Read the model definition and answer for the solid it produces. Units are mm, in the model's axes. Give positions to 0.01 mm unless a question says otherwise; leave off trailing zeros. Write each loop counter-clockwise with the first axis right and the second up, starting at its lowest first coordinate (ties: lowest second). Pieces come first, ordered by that corner, then holes.
```python
from build123d import *

# Parameters (mm, degrees)
SKETCH1_W           = 25.4
SKETCH1_H           = 25.4
SKETCH1_W_2         = 20.32
SKETCH1_H_2         = 20.32
BOSS_EXTRUDE2_DEPTH = 368.3
CUT_EXTRUDE1_DEPTH  = 370.393205135
SKETCH3_R           = 3.175
CUT_EXTRUDE2_DEPTH  = 370.393205135


with BuildPart() as part:
    # Sketch1 → Boss-Extrude2 (new body)
    with BuildSketch(Plane.XY):
        Rectangle(SKETCH1_W, SKETCH1_H)
        Rectangle(SKETCH1_W_2, SKETCH1_H_2, mode=Mode.SUBTRACT)
    extrude(amount=BOSS_EXTRUDE2_DEPTH)

    # Sketch2 → Cut-Extrude1 (cut, through all)
    with BuildSketch(Plane(origin=(0, 12.7, 0), x_dir=(1, 0, 0), z_dir=(0, 1, 0))):
        Polygon((-12.7, -368.3), (12.7, -353.635303163), (12.7, -368.3), align=None)
        Polygon((12.7, 0), (-12.7, 0), (12.7, -14.664696837), align=None)
    extrude(amount=-CUT_EXTRUDE1_DEPTH, mode=Mode.SUBTRACT)

    # Sketch3 → Cut-Extrude2 (cut, through all)
    with BuildSketch(Plane(origin=(0, 12.7, 0), x_dir=(1, 0, 0), z_dir=(0, 1, 0))):
        with Locations(Location((0, -184.15, 0), (0, 0, 270))):
            Circle(SKETCH3_R)
        with Locations(Location((0, -171.45, 0), (0, 0, 270))):
            Circle(SKETCH3_R)
        with Locations(Location((0, -158.75, 0), (0, 0, 270))):
            Circle(SKETCH3_R)
        with Locations((0, -209.55)):
            Circle(SKETCH3_R)
        with Locations((0, -196.85)):
            Circle(SKETCH3_R)
        with Locations(Location((0, -349.25, 0), (0, 0, 270))):
            Circle(SKETCH3_R)
        with Locations(Location((0, -336.55, 0), (0, 0, 270))):
            Circle(SKETCH3_R)
        with Locations(Location((0, -323.85, 0), (0, 0, 270))):
            Circle(SKETCH3_R)
        with Locations(Location((0, -311.15, 0), (0, 0, 270))):
            Circle(SKETCH3_R)
        with Locations(Location((0, -298.45, 0), (0, 0, 270))):
            Circle(SKETCH3_R)
        with Locations((0, -69.85)):
            Circle(SKETCH3_R)
        with Locations((0, -57.15)):
            Circle(SKETCH3_R)
        with Locations((0, -44.45)):
            Circle(SKETCH3_R)
        with Locations((0, -31.75)):
            Circle(SKETCH3_R)
        with Locations((0, -19.05)):
            Circle(SKETCH3_R)
    extrude(amount=-CUT_EXTRUDE2_DEPTH, mode=Mode.SUBTRACT)


solid = part.part
```
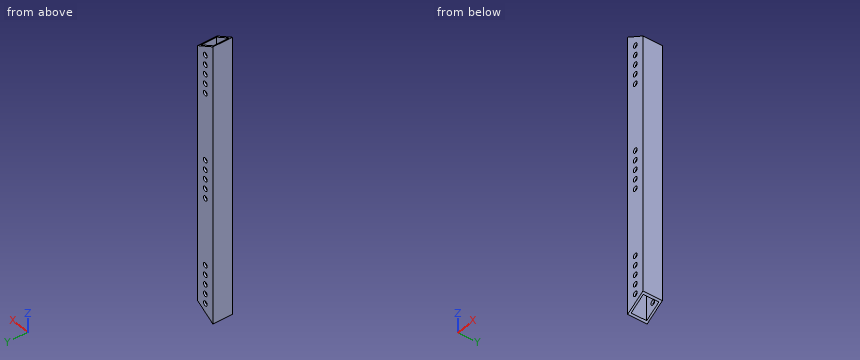
Item 1: Section B-B (z = 184.15) is taken. Write down the section's boundary in (x, y) (3 decimals), and give its area (3 significant figures).
Result set:
outline: (-12.7, -12.7) - (-3.175, -12.7) - (-3.175, -10.16) - (-10.16, -10.16) - (-10.16, 10.16) - (-3.175, 10.16) - (-3.175, 12.7) - (-12.7, 12.7) - close; (3.175, -12.7) - (12.7, -12.7) - (12.7, 12.7) - (3.175, 12.7) - (3.175, 10.16) - (10.16, 10.16) - (10.16, -10.16) - (3.175, -10.16) - close
area: 200 mm2
Item 2: Section C-C (z = 121.5) is taken. Write down the section's boundary in (x, y), and give its area (3 significant figures).
Result set:
outline: (-12.7, -12.7) - (12.7, -12.7) - (12.7, 12.7) - (-12.7, 12.7) - close; hole (-10.16, -10.16) - (10.16, -10.16) - (10.16, 10.16) - (-10.16, 10.16) - close
area: 232 mm2
Item 3: Each of these flat-tipped pins is pushed along its axis until it touches: pin 1 Ø4 at (x, z) = (0, 196.85) entering from -Y; pin 2 Ø3 at (x, y) = (-5, 9) entering from -Z. Where does it stop, or does it pass through?
Result set:
pin 1: passes through
pin 2: stops at z = 3.9
Item 4: Section D-D (x = -7) is taken. Write down the section's boundary in (y, z), and give its area (3 significant figures).
Result set:
outline: (-12.7, 3.29) - (-10.16, 3.29) - (-10.16, 365.01) - (-12.7, 365.01) - close; (10.16, 3.29) - (12.7, 3.29) - (12.7, 365.01) - (10.16, 365.01) - close
area: 1,840 mm2
Item 5: Find the intervals of material crossed by line 1 along Y through (x, z) = (-5.5, 291.5); line 2 along X through (y, z) = (-10.85, 31.75) (3 decimals), in increasing order.
Result set:
line 1: y = -12.7 to -10.16, 10.16 to 12.7
line 2: x = -12.7 to -3.175, 3.175 to 12.7
Item 6: Section A-A (y = 0) is taken. Write down the section's boundary in (x, z), and give its area (3 significant figures).
Result set:
outline: (-12.7, 0) - (-10.16, 1.47) - (-10.16, 366.83) - (-12.7, 368.3) - close; (10.16, 13.2) - (12.7, 14.66) - (12.7, 353.64) - (10.16, 355.1) - close
area: 1,800 mm2
